Autodesk Inventor part; units mm, degrees
ref_plane "YZ Plane" through (0, 0, 0) normal (1, 0, 0) x (0, 1, 0)
ref_plane "XZ Plane" through (0, 0, 0) normal (0, 1, 0) x (-1, 0, 0)
ref_plane "XY Plane" through (0, 0, 0) normal (0, 0, 1) x (1, 0, 0)
sketch "Skizze1" plane through (0, 0, 0) normal (0, 1, 0) x (-1, 0, 0)
  line L0 (0, 0) -> (60, 0)
  line L1 (60, 0) -> (60, -60)
  line L2 (60, -60) -> (0, -60)
  line L3 (0, -60) -> (0, 0)
  dimension "d0" = 60
  dimension "d1" = 60
extrude "Extrusion1" add sketch "Skizze1" along normal blind 6
sketch "m" plane through (0, 6, 0) normal (0, 1, 0) x (1, 0, 0)
  line L0 (-60, 0) -> (0, 0)
  line L1 (-60, 60) -> (-60, 0)
  line L2 (0, 0) -> (0, 60)
  line L3 (0, 60) -> (-60, 60)
  point P0 (-50, 3)
  point P1 (-10, 3)
  point P2 (-50, 57)
  point P3 (-10, 57)
  dimension "d4" = 3
  dimension "d5" = 10
  dimension "d6" = 10
  dimension "d7" = 3
hole "Bohrung1" at (-50, 6, -3) at (-10, 6, -3) at (-50, 6, -57) at (-10, 6, -57) direction (0, -1, 0) diameter 2.5 depth 10 tip angle 118
chamfer "Fase1" distance 1 angle 45 4 edges at (-10, 6, -58.25) (-50, 6, -58.25) (-10, 6, -4.25) (-50, 6, -4.25)
properties part number "AkkuHaltBoden"
Read the model definition and answer for the solid it produces. Units are mm, in the model's axes. Round coordinates to 2 decimals unless told otherwise and drop trailing zeros. Write each loop counter-clockwise with the first axis right and the second up, starting at its lowest first coordinate (ties: lowest second). Pieces come first, ordered by that corner, then holes.
1. Straight lines are drawn through the part: L1, parallel to Z at x = -10, y = 3; L2, parallel to X at y = 2.85, z = -3; L3, parallel to X at y = 5.65, z = -56. For each, find the intervals that lie inside material, in ascending order.
2. Determine the mould class of faces 1 (the face through (-30, 6, -30)), 2 (the face through (-11.054, 2.465, -2.328)), 3 (the face through (-50.38, 2.46, -55.81)), 4 (the face through (-30, 3, 0)) for opening direction Z: pulls with the +Z half, pulls with the -Z half, needs draft (parallel to the pull), parting line crosses it, or undercut.
3. Given pin 1 Ø2 at (x, z) = (-50, -3) entering from -Y, flat-ended and moving along its own axis, determine where the tip first touches the part or whether it passes through.
4. The part is cut by section A-A, the plane z = -57. Determine the outline of the cut face in (x, y), then the cut area to 3 significant figures.
5. The part is cut by section B-B, the plane x = -10. Determine the outline of the cut face in (y, z).
Values:
1. L1: z = -60 to -58.25, -55.75 to -4.25, -1.75 to 0
1. L2: x = -60 to -51.25, -48.75 to -11.25, -8.75 to 0
1. L3: x = -60 to -51.62, -48.38 to -11.62, -8.38 to 0
2. face 1: needs draft
2. face 2: undercut
2. face 3: undercut
2. face 4: pulls with the +Z half
3. pin 1: passes through
4. outline: (-60, 0) - (-51.25, 0) - (-51.25, 5) - (-52.25, 6) - (-60, 6) - close; (-48.75, 0) - (-11.25, 0) - (-11.25, 5) - (-12.25, 6) - (-47.75, 6) - (-48.75, 5) - close; (-8.75, 0) - (0, 0) - (0, 6) - (-7.75, 6) - (-8.75, 5) - close
4. area: 328 mm2
5. outline: (0, -60) - (6, -60) - (6, -59.25) - (5, -58.25) - (0, -58.25) - close; (0, -55.75) - (5, -55.75) - (6, -54.75) - (6, -5.25) - (5, -4.25) - (0, -4.25) - close; (0, -1.75) - (5, -1.75) - (6, -0.75) - (6, 0) - (0, 0) - close
